Model file for the job. Use its own axes, mm. Face numbers are marked on the shaded views. A direction names the side the tool comes from. Give positions to 0.01 mm unless a question says otherwise; leave off trailing zeros. Write each loop counter-clockwise with the first axis right and the second up, starting at its lowest first coordinate (ties: lowest second). Pieces come first, ordered by that corner, then holes. Notation, with made-up numbers: M 25,81.25 L 75,81.25 A22 ccw 75,110.25 Z; hole C 7.5,-25 d6. An arc over 180 degrees is marked long. Answer as a JSON object with one key per item and string values. Group by question number.
Autodesk Inventor part; units mm, degrees
ref_plane "YZ Plane" through (0, 0, 0) normal (1, 0, 0) x (0, 1, 0)
ref_plane "XZ Plane" through (0, 0, 0) normal (0, 1, 0) x (-1, 0, 0)
ref_plane "XY Plane" through (0, 0, 0) normal (0, 0, 1) x (1, 0, 0)
sketch "Sketch1" plane through (0, 0, 0) normal (0, 0, 1) x (1, 0, 0)
  circle A0 centre (0, 0) radius 3.55
  line L0 (-2.2753, 2.725) -> (2.2753, 2.725)
  line L1 (2.2753, -2.725) -> (-2.2753, -2.725)
  circle A1 centre (0, 0) radius 4.25
  dimension "d0" = 7.1
  dimension "d1" = 5.45
  dimension "d2" = 8.5
extrude "Extrusion1" add sketch "Sketch1" along normal blind 1.25 contours L0 A0 | A0 L1 | A1
sketch "Sketch4" plane through (0, 0, 1.25) normal (0, 0, 1) x (1, 0, 0)
  circle A0 centre (0, 0) radius 4.25
  circle A1 centre (0, 0) radius 1
  dimension "d7" = 2
extrude "Extrusion2" add sketch "Sketch4" along normal blind 1.25
fillet "Fillet1" radius 1 1 edges at (-4.25, 0, 2.5)
properties part number "EncoderV2CAP"
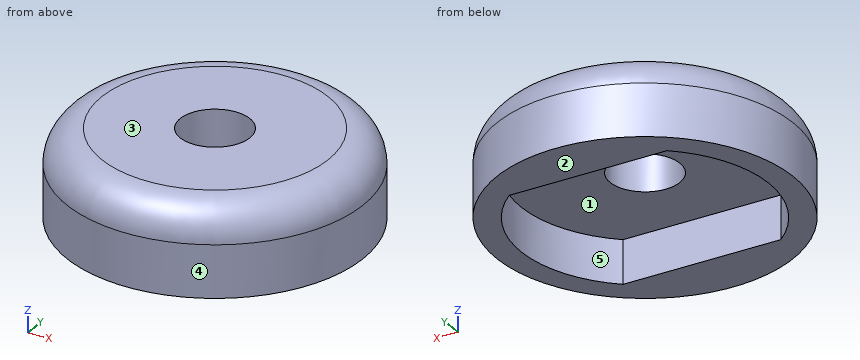
Q1. Slice it at D-D, the plane z = 1.9. Write the cut outline in (x, y), then the cut area to 3 significant figures.
Q2. Slice it at A-A, the plane x = 0. Write the cut outline in (y, z) (3 decimals).
Q3. Wall check: L1, parallel to Y at x = 0, z = 1.55; L2, parallel to Z at x = 2.5, y = -2; L3, parallel to Y at x = -1.5, z = 0.55 (1 decimal). Give the ranges that are in metal, low to high.
Q4. Slice it at B-B, the plane y = 0. Write the cut outline in (x, z), then the cut area to 3 significant figures.
Q5. Drop flat-ended pins along their axis: P1, Ø1.8, axis at x = 0, y = 0, coming from the +Z side; P2, Ø0.6, axis at x = -0.5, z = 0.5, coming from the -Y side; P3, Ø1, axis at x = 1.5, z = 2, coming from the -Y side; P4, Ø1, axis at x = -1, y = -1, coming from the -Z side. Give the stop position or say it passes through.
Q6. 3-axis set-ups, long thin cutter, end or side, ignore diameter. For the marked faces 1 and 2: which of +Z, -Z, +X, -X, +Y, -Y reach the whole face in a straight line?
Q7. Slice it at C-C, the plane z = 0.2. Write the cut outline in (x, y) (3 decimals), then the cut area to 3 significant figures.
Q8. Two-plate mould, pull along Y, no slides. Class the marked faces 3, 4 and 5: +Y half, -Y half, draft (parallel to the pull), parting line (faces both ways), or undercut.
Solved:
{
 "1": {"outline": "C 0,0 d8.33; hole C 0,0 d2", "area": "51.4 mm²"},
 "2": {"outline": "M -4.25,0 L -2.725,0 L -2.725,1.25 L -1,1.25 L -1,2.5 L -3.25,2.5 A1 ccw -4.25,1.5 Z; M 1,1.25 L 2.725,1.25 L 2.725,0 L 4.25,0 L 4.25,1.5 A1 ccw 3.25,2.5 L 1,2.5 Z"},
 "3": {"L1": "y = -4.25 to -1, 1 to 4.25", "L2": "z = 1.25 to 2.5", "L3": "y = -4 to -2.7, 2.7 to 4"},
 "4": {"outline": "M -4.25,0 L -3.55,0 L -3.55,1.25 L -1,1.25 L -1,2.5 L -3.25,2.5 A1 ccw -4.25,1.5 Z; M 1,1.25 L 3.55,1.25 L 3.55,0 L 4.25,0 L 4.25,1.5 A1 ccw 3.25,2.5 L 1,2.5 Z", "area": "9.45 mm²"},
 "5": {"P1": "passes through", "P2": "stops at y = -4.25", "P3": "stops at y = -4.08", "P4": "stops at z = 1.25"},
 "6": {"face 1": "-Z", "face 2": "-Z, +X, -X, +Y, -Y"},
 "7": {"outline": "C 0,0 d8.5; hole M -2.275,-2.725 L 2.275,-2.725 A3.55 ccw 2.275,2.725 L -2.275,2.725 A3.55 ccw Z", "area": "22.3 mm²"},
 "8": {"face 3": "draft", "face 4": "parting line", "face 5": "undercut"}
}
